Part model, mm, in its own coordinate system. A direction names the side the tool comes from. Give positions to 0.01 mm unless a question says otherwise; leave off trailing zeros. Loops run counter-clockwise (first coordinate to the right, second up) from the corner with the lowest first, then second, coordinate; pieces in that order, holes last. Notation, with made-up numbers: (18.25, 46) -> (33.25, 46) arc R26 cw to (33.25, 61) -> close; hole circle Ø1 at (50.5, 67.5). An arc over 180 degrees is marked (long way). One line per question, with ' | ' between items.
```python
from build123d import *

# Parameters (mm, degrees)
F0_R     = 12.7
F1_DEPTH = 50.8
F3_DEPTH = 3.175
F5_DEPTH = 3.175
F7_D     = 6.35


with BuildPart() as f1:
    # F0 (on Front) → F1 (new body)
    with BuildSketch(Plane.XZ):
        Circle(F0_R)
    extrude(amount=F1_DEPTH)

    # F2 (on Right) → F3 (join, symmetric)
    with BuildSketch(Plane.YZ):
        Polygon((0, 0), (0, 25.4), (-50.8, 25.4), (-50.8, -25.4), (0, -25.4), align=None)
    extrude(amount=F3_DEPTH, both=True)

    # F4 (on Top) → F5 (join, symmetric)
    with BuildSketch(Plane.XY):
        Polygon((0, 0), (-25.4, 0), (-25.4, -50.8), (25.4, -50.8), (25.4, 0), align=None)
    extrude(amount=F5_DEPTH, both=True)

    # F7 (through all)
    with Locations(Plane(origin=(0, 0, 0), x_dir=(-1, 0, 0), z_dir=(0, 1, 0))):
        with Locations((0, 0)):
            Hole(F7_D / 2)


solid = f1.part
```
1) Pin check, flat tips, straight feed: P1, Ø1, axis at y = -43, z = 7, coming from the +X side; P2, Ø4, axis at y = -33.5, z = -20, coming from the +X side (3 decimals); P3, Ø4, axis at y = -20, z = -18.5, coming from the -X side (3 decimals). Stop position of each tip, or through.
Found:
P1: x = 10.91 | P2: x = 3.175 | P3: x = -3.175
2) Tool access for faces 1 (the flat face through (0, -26, -25.4)), 2 (the flat face through (-19, -25, -3.175)), 3 (the flat face through (3.175, -26, -19)), 4 (the flat face through (19, -25, 3.175)), 5 (the flat face through (-3.175, -26, 19)): list every direction of +Z, -Z, +X, -X, +Y, -Y with a clear straight run to the whole face (end or side of a thin tool).
Found:
face 1: -Z, +X, -X, +Y, -Y | face 2: -Z, -X, +Y, -Y | face 3: -Z, +X, +Y, -Y | face 4: +Z, +X, +Y, -Y | face 5: +Z, -X, +Y, -Y
3) Saw through at C-C (z = 0). Give the cut face in (x, y) (3 decimals), and give its area (3 significant figures).
Found:
outline: (-25.4, -50.8) -> (-3.175, -50.8) -> (-3.175, 0) -> (-25.4, 0) -> close; (3.175, -50.8) -> (25.4, -50.8) -> (25.4, 0) -> (3.175, 0) -> close | area: 2,260 mm2
4) Drill centre lines: line 1 (Z direction, x = 0, y = -19) (3 decimals); line 2 (Z direction, x = 21, y = -40) (3 decimals); line 3 (X direction, y = -27.5, z = 1.5). Where is each one in solid material? Low to high.
Found:
line 1: -25.4 to -3.175, 3.175 to 25.4 | line 2: -3.175 to 3.175 | line 3: -25.4 to -2.8, 2.8 to 25.4
5) Saw through at D-D (x = 19). Give the cut face in (y, z) (3 decimals), and give its area (3 significant figures).
Found:
outline: (-50.8, -3.175) -> (0, -3.175) -> (0, 3.175) -> (-50.8, 3.175) -> close | area: 323 mm2
6) Saw through at B-B (y = -40.5). Give the cut face in (x, z) (3 decimals), and give its area (3 significant figures).
Found:
outline: (-25.4, -3.175) -> (-12.297, -3.175) arc R12.7 ccw to (-3.175, -12.297) -> (-3.175, -25.4) -> (3.175, -25.4) -> (3.175, -12.297) arc R12.7 ccw to (12.297, -3.175) -> (25.4, -3.175) -> (25.4, 3.175) -> (12.297, 3.175) arc R12.7 ccw to (3.175, 12.297) -> (3.175, 25.4) -> (-3.175, 25.4) -> (-3.175, 12.297) arc R12.7 ccw to (-12.297, 3.175) -> (-25.4, 3.175) -> close; hole circle Ø6.35 at (0, 0) | area: 801 mm2
7) Saw through at A-A (x = 0). Give the cut face in (y, z) (3 decimals), and give its area (3 significant figures).
Found:
outline: (-50.8, -25.4) -> (0, -25.4) -> (0, -3.175) -> (-50.8, -3.175) -> close; (-50.8, 3.175) -> (0, 3.175) -> (0, 25.4) -> (-50.8, 25.4) -> close | area: 2,260 mm2
